```python
from build123d import *

# Parameters (mm, degrees)
SKETCH001_R  = 2
PAD_DEPTH    = 6
SKETCH_W     = 25
SKETCH_H     = 8.532326
SKETCH_R     = 2
PAD001_DEPTH = 4
SKETCH002_R  = 8
POCKET_DEPTH = 25.001


with BuildPart() as part:
    # Sketch001 → Pad (new body)
    with BuildSketch(Plane.XY):
        with BuildLine():
            Line((0, -0.513451), (12.5, -0.513451))
            Line((12.5, -0.513451), (12.5, 8.018875))
            Line((12.5, 8.018875), (5.444822, 8.018875))
            Line((5.444822, 8.018875), (2.947073, 22.018734))
            ThreePointArc((2.947073, 22.018734), (1.921936, 23.788122), (0, 24.486549))
            ThreePointArc((0, 24.486549), (-1.921936, 23.788122), (-2.947073, 22.018734))
            Line((-5.444822, 8.018875), (-2.947073, 22.018734))
            Line((-12.5, 8.018875), (-5.444822, 8.018875))
            Line((-12.5, -0.513451), (-12.5, 8.018875))
            Line((0, -0.513451), (-12.5, -0.513451))
        make_face()
        with Locations((-7.553649, 3.816244)):
            Circle(SKETCH001_R, mode=Mode.SUBTRACT)
        with Locations((7.553649, 3.816244)):
            Circle(SKETCH001_R, mode=Mode.SUBTRACT)
    extrude(amount=PAD_DEPTH)

    # Sketch → Pad001 (new body)
    with BuildSketch(Plane.XY.offset(6)):
        with Locations((0, 3.752712)):
            Rectangle(SKETCH_W, SKETCH_H)
        with Locations((-7.553649, 3.816244)):
            Circle(SKETCH_R, mode=Mode.SUBTRACT)
        with Locations((7.553649, 3.816244)):
            Circle(SKETCH_R, mode=Mode.SUBTRACT)
    extrude(amount=PAD001_DEPTH)

    # Sketch002 → Pocket (cut, through all)
    with BuildSketch(Plane.YZ.offset(12.5)):
        with Locations((15.447758, 10.107347)):
            Circle(SKETCH002_R)
    extrude(amount=-POCKET_DEPTH, mode=Mode.SUBTRACT)


solid = part.part
```
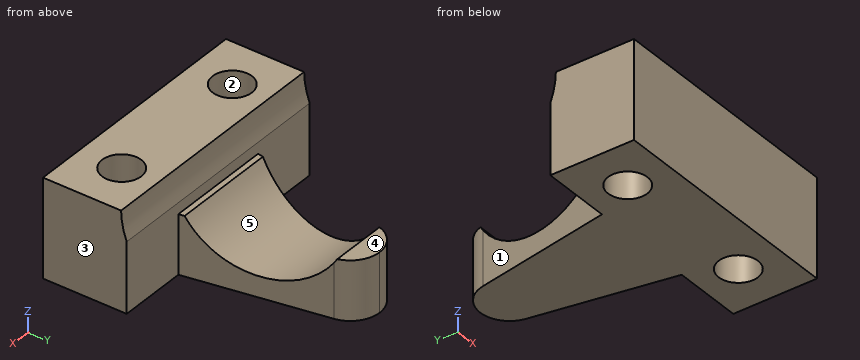
Check sheet for the modelled part. Datum: model origin and axes. Units: mm. Face numbers are marked on the shaded views. A direction names the side the tool comes from. Coordinates: 2 decimals unless noted, no trailing zeros. Loops run counter-clockwise (first coordinate to the right, second up) from the corner with the lowest first, then second, coordinate; pieces in that order, holes last.
1) Access from +Z, -Z, +X, -X, +Y, -Y to the whole of each face (thin tool, end or side, straight path). Record for the marked faces 4 and 5.
2) Sectioned sample at D-D (x = -1.5). Record the boundary of the cut face in (y, z).
3) Material ranges on probe 1 along X at (y, z) = (3, 1.25); probe 2 along X at (y, z) = (5.5, 1.5); probe 3 along Y at (x, z) = (7.75, 3.5), recorded low to high.
4) Release check for a two-part mould opening along Y. For the marked faces 1, 2 and 3 record: released by +Y, released by -Y, zero draft, split by the parting line, or undercut.
5) Gauge pin test, flat ends, axial feed: pin 1 (1.7 mm diameter, centred on x = 1, y = 24, fed in from +Z); pin 2 (6 mm diameter, centred on x = 5.5, y = 15.5, fed in from +Z); pin 3 (2 mm diameter, centred on x = 0.5, y = 17, fed in from +Z). Record the tip position at first contact, or that the pin passes through.
6) Sectioned sample at A-A (z = 3.25). Record the boundary of the cut face in (x, y).
7) Sectioned sample at B-B (x = 6.25). Record the boundary of the cut face in (y, z), and give its area (3 significant figures).
8) Sectioned sample at C-C (z = 1). Record the boundary of the cut face in (x, y), and give its area (3 significant figures).
Check sheet entries:
1. face 4: +Z, +X, -X, +Y
1. face 5: +Z, +X, -X
2. outline: (-0.51, 0) - (24.08, 0) - (24.08, 6) - (22.31, 6) arc R8 cw to (8.58, 6) - (8.02, 6) - (8.02, 7.14) arc R8 cw to (7.45, 10) - (-0.51, 10) - close
3. probe 1: x = -12.5 to -9.38, -5.73 to 5.73, 9.38 to 12.5
3. probe 2: x = -12.5 to -8.63, -6.47 to 6.47, 8.63 to 12.5
3. probe 3: y = -0.51 to 1.83, 5.81 to 8.02
4. face 1: released by +Y
4. face 2: undercut
4. face 3: zero draft
5. pin 1: stops at z = 6
5. pin 2: stops at z = 2.62
5. pin 3: stops at z = 2.53
6. outline: (-12.5, -0.51) - (12.5, -0.51) - (12.5, 8.02) - (5.44, 8.02) - (4.85, 11.33) - (-4.85, 11.33) - (-5.44, 8.02) - (-12.5, 8.02) - close; (-3.38, 19.57) - (3.38, 19.57) - (2.95, 22.02) arc R2.99 ccw to (0, 24.49) arc R2.99 ccw to (-2.95, 22.02) - close; hole circle Ø4 at (-7.55, 3.82); hole circle Ø4 at (7.55, 3.82)
7. outline: (-0.51, 0) - (2.3, 0) - (2.3, 10) - (-0.51, 10) - close; (5.33, 0) - (8.02, 0) - (8.02, 7.14) arc R8 cw to (7.45, 10) - (5.33, 10) - close
7. area: 53.9 mm2
8. outline: (-12.5, -0.51) - (12.5, -0.51) - (12.5, 8.02) - (5.44, 8.02) - (2.95, 22.02) arc R2.99 ccw to (0, 24.49) arc R2.99 ccw to (-2.95, 22.02) - (-5.44, 8.02) - (-12.5, 8.02) - close; hole circle Ø4 at (-7.55, 3.82); hole circle Ø4 at (7.55, 3.82)
8. area: 317 mm2
